The model under review builds one solid part; all positions refer to its coordinate system, in mm. Face numbers are marked on the shaded views. A direction names the side the tool comes from. Round coordinates to 2 decimals unless told otherwise and drop trailing zeros. Write each loop counter-clockwise with the first axis right and the second up, starting at its lowest first coordinate (ties: lowest second). Pieces come first, ordered by that corner, then holes. Notation, with made-up numbers: (52, 7.25) - (92, 7.25) arc R24 cw to (92, 34.25) - close; hole circle Ø4 at (-14, 76). An arc over 180 degrees is marked (long way). Write each question's results on one line, items separated by ' | '.
Autodesk Inventor part; units mm, degrees
ref_plane "Work Plane1" through (0, 0, 0) normal (0, -1, 0) x (1, 0, 0)
ref_plane "YZ Plane" through (0, 0, 0) normal (1, 0, 0) x (0, 1, 0)
ref_plane "XZ Plane" through (0, 0, 0) normal (0, 1, 0) x (-1, 0, 0)
ref_plane "Work Plane1" through (0, 0, 0) normal (0, -1, 0) x (1, 0, 0)
sketch "Sketch1" plane through (0, 0, 0) normal (0, -1, 0) x (1, 0, 0)
  circle A0 centre (0, 0) radius 52
  circle A1 centre (0, 0) radius 62
  circle A2 centre (0, 0) radius 52
  dimension "d1" = 10
extrude "Extrusion1" add sketch "Sketch1" against normal blind 25
sketch "Sketch3" plane through (0, 0, 0) normal (0, -1, 0) x (1, 0, 0)
  circle A0 centre (0, 0) radius 62
  circle A1 centre (0, 0) radius 50
  circle A2 centre (0, 0) radius 52
  dimension "d9" = 124
  dimension "d10" = 2
extrude "Extrusion3" add sketch "Sketch3" along normal blind 2 contours A0 | A2
sketch "Sketch4" plane through (0, -2, 0) normal (0, -1, 0) x (1, 0, 0)
  circle A0 centre (0, 0) radius 62 construction
  line L0 (-62, 0) -> (62, 0) construction
  line L1 (0, 62) -> (0, -62) construction
ref_plane "Work Plane2" through (-62, -2, 0) normal (0, 0, 1) x (1, 0, 0)
sketch "Sketch5" plane through (-62, -2, 0) normal (0, 0, 1) x (1, 0, 0)
  line L0 (0, 0) -> (124, 0) construction
  line L1 (62, 0) -> (62, -30) construction
  line L2 (62, 0) -> (62, -30) construction
  line L3 (82, -30) -> (124, 0) construction
  line L4 (62, 0) -> (62, -30) construction
  line L5 (62, 0) -> (62, -30)
  line L6 (82, -30) -> (124, 0)
  line L7 (62, 0) -> (124, 0)
  line L8 (82, -30) -> (62, -30)
  point P0 (62, 2)
  dimension "d14" = 20
  dimension "d23" = 30
revolve "Revolution1" add sketch "Sketch5" angle 360 about axis through (0, -2, 0) along (0, -1, 0)
shell "Shell1" thickness 2 removed faces 2 at (9.39, -2, -8.8667) at (-4.4202, -32, 2.9181)
fillet "Fillet2" radius 5 1 edges at (-62, 25, 0)
sketch "Sketch6" plane through (0, -32, 0) normal (0, -1, 0) x (1, 0, 0)
  circle A0 centre (0, 0) radius 20
  circle A1 centre (0, 0) radius 17.2734
  point P0 (0, 0)
extrude "Extrusion4" add sketch "Sketch6" along normal blind 10
sketch "Sketch7" plane through (-62, -2, 0) normal (0, 0, 1) x (1, 0, 0)
  line L0 (116, 0) -> (8, 0) construction
  line L1 (62, 0) -> (62, -68.8676) construction
  line L2 (62, -68.8676) -> (62, 58.2557) construction
  point P0 (62, 2)
sketch "Sketch8" plane through (0, -42, 0) normal (0, -1, 0) x (1, 0, 0)
  circle A0 centre (0, 0) radius 17.2734 construction
  circle A1 centre (0, 0) radius 20 construction
  point P0 (0, 0)
  dimension "d21" = 34.5467
  dimension "d22" = 40
properties part number "JarCone"
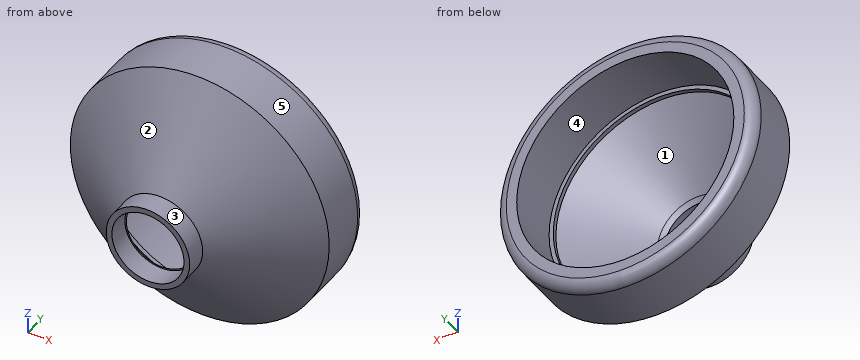
Q1. Tool access review of the marked faces 3, 4 and 5: name each direction out of +Z, -Z, +X, -X, +Y, -Y from which nothing blocks a thin tool from reaching the whole face with its end or side.
Evaluation:
face 3: -Y | face 4: +Y | face 5: +Y, -Y
Q2. We need section A-A (y = 12.5). State the section outline as (x, z) points.
Evaluation:
outline: circle Ø124 at (0, 0); circle Ø108 at (0, 0); hole circle Ø120 at (0, 0); hole circle Ø104 at (0, 0)
Q3. The part is to be moulded in two halves that separate along X. For the marked faces 1 and 2, say which applies: released by +X, released by -X, zero draft, split by the parting line, or undercut.
Evaluation:
face 1: undercut | face 2: split by the parting line
Q4. Insertion check: P1, Ø6, axis at y = -26.5, z = -14.5, coming from the -X side; P2, Ø20.5, axis at x = 0, z = 0, coming from the +Y side; P3, Ø6, axis at x = 8.5, z = -25.5, coming from the -Y side; P4, Ø6, axis at x = -38.5, y = 12, coming from the +Z side. Each pin has a flat end and moves straight along its axis. Give the tip position at first contact, or say it passes through.
Evaluation:
P1: stops at x = -28.64 | P2: passes through | P3: stops at y = -29.23 | P4: stops at z = 50.83
Q5. For probe 1 along Z at (x, y) = (0, 13.5); probe 2 along X at (y, z) = (11, -11.5); probe 3 along Z at (x, y) = (-14.5, 6), list the stretches that pass through material, from the lowest coordinate up.
Evaluation:
probe 1: z = -62 to -60, -54 to -52, 52 to 54, 60 to 62 | probe 2: x = -60.92 to -58.89, -52.76 to -50.71, 50.71 to 52.76, 58.89 to 60.92 | probe 3: z = -60.28 to -58.22, -52.02 to -49.94, 49.94 to 52.02, 58.22 to 60.28
